Design review of the part shown in the three views and the two pictorial views. Dimensions are in mm from the part's minimum x, y and z. A direction names the side the tool comes from. Round coordinates to 2 decimals unless told otherwise and drop trailing zeros. Write each loop counter-clockwise with the first axis right and the second up, starting at its lowest first coordinate (ties: lowest second). Pieces come first, ordered by that corner, then holes. Notation, with made-up numbers: (38, 87) - (91, 87) arc R23 ccw to (91, 106) - close; hole circle Ø11 at (32, -32). An arc over 180 degrees is marked (long way). Use one line per item in the form item = value.
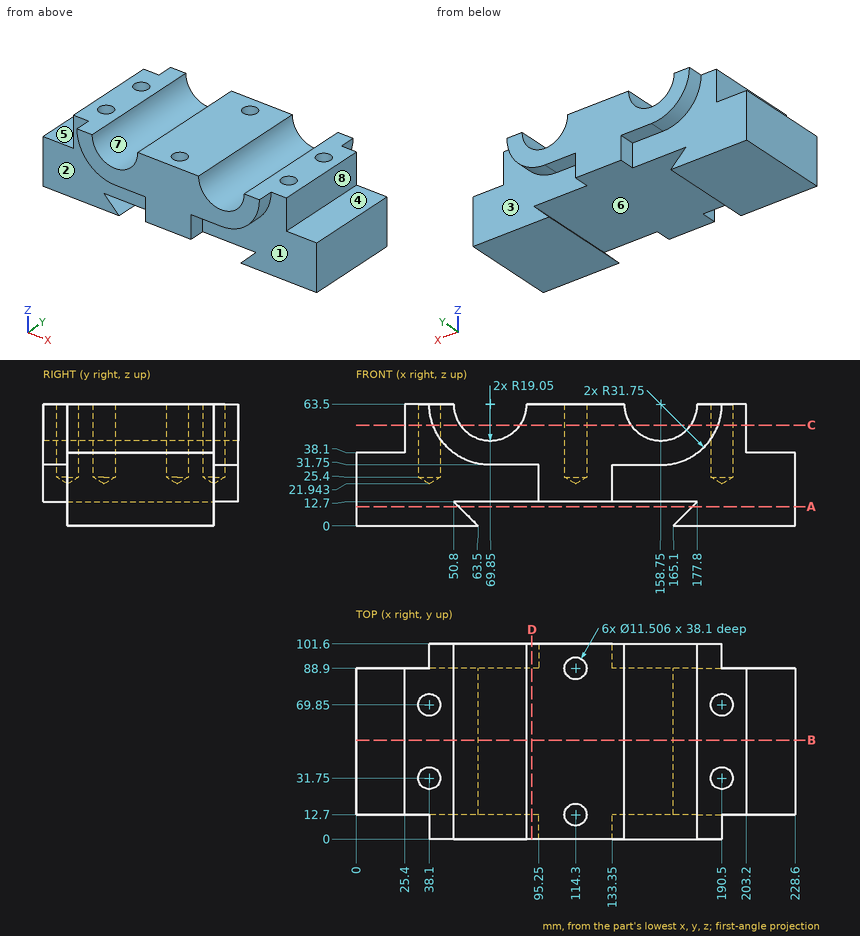
Q1. Draft analysis for pull direction Z (two halves, no side actions). For the marked faces 6, 7 and 8, state which applies: released by +Z, released by -Z, zero draft, split by the parting line, or undercut.
Calculated:
face_6 = undercut
face_7 = released by +Z
face_8 = zero draft
Q2. We need section D-D on x = 91.5. Write out the cut boundary in (y, z), then the cut area to 3 significant figures.
Calculated:
outline = (0, 31.75) - (12.7, 31.75) - (12.7, 12.7) - (88.9, 12.7) - (88.9, 31.75) - (101.6, 31.75) - (101.6, 63.5) - (0, 63.5) - close
area = 4,680 mm2
Q3. We need section A-A on z = 10. Write out the cut boundary in (x, y).
Calculated:
outline = (0, 12.7) - (53.5, 12.7) - (53.5, 88.9) - (0, 88.9) - close; (175.1, 12.7) - (228.6, 12.7) - (228.6, 88.9) - (175.1, 88.9) - close
Q4. Machinability: for the marked faces 1, 2, 3, 4 and 5, which of the approach directions +Z, -Z, +X, -X, +Y, -Y give a long, thin tool a straight path to every point of the face, cutting with its end or side? Answer none if there is none.
Calculated:
face_1 = -Z, +X, -Y
face_2 = -Z, -X, -Y
face_3 = -Z, +X, +Y
face_4 = +Z, +X, +Y, -Y
face_5 = +Z, -X, +Y, -Y
Q5. For P1, Ø4, axis at y = 4.5, z = 26, coming from the -X side; P2, Ø12.5, axis at x = 17, y = 57.5, coming from the +Z side; P3, Ø4, axis at x = 81.5, y = 7, coming from the -Z side, all flat-tipped, find the tip position at first contact; note any pin that passes through.
Calculated:
P1 = 95.25
P2 = 38.1
P3 = 31.75
Q6. To check wall thickness, follow line 1 along Y through (x, z) = (38, 41); line 2 along Y through (x, z) = (114, 44) (1 decimal); line 3 along X through (y, z) = (31, 34.5). State the ranges of each line that lie inside material, in increasing order. Write a range as from..to.
Calculated:
line_1 = 12.7..26, 37.5..64.1, 75.6..88.9
line_2 = 0..7, 18.4..83.2, 94.6..101.6
line_3 = 0..32.4, 43.8..184.8, 196.2..228.6
Q7. We need section B-B on y = 51.5. Write out the cut boundary in (x, z).
Calculated:
outline = (0, 0) - (63.5, 0) - (50.8, 12.7) - (177.8, 12.7) - (165.1, 0) - (228.6, 0) - (228.6, 38.1) - (203.2, 38.1) - (203.2, 63.5) - (177.8, 63.5) arc R19.05 cw to (139.7, 63.5) - (88.9, 63.5) arc R19.05 cw to (50.8, 63.5) - (25.4, 63.5) - (25.4, 38.1) - (0, 38.1) - close
Q8. We need section C-C on z = 52.5. State how many separate pieces and enclosed holes the cut face has, then the cut area to 3 significant figures.
Calculated:
separate_pieces = 3
enclosed_holes = 6
area = 10,400 mm2
